Can you work these out from the drawing? Everything is in mm from the part's minimum corner. A direction names the side the tool comes from. Coordinates: 2 decimals unless noted, no trailing zeros. Order: outer loops, then holes, each group sorted by start corner. A loop starts at its lowest first (then second) coordinate and runs counter-clockwise, first axis right, second up. Notation, with made-up numbers: (76, -37) -> (134, -37) arc R9 cw to (134, -22) -> close; hole circle Ø4 at (89.5, -27). An arc over 180 degrees is marked (long way). Answer in a Markdown table with one row per item.
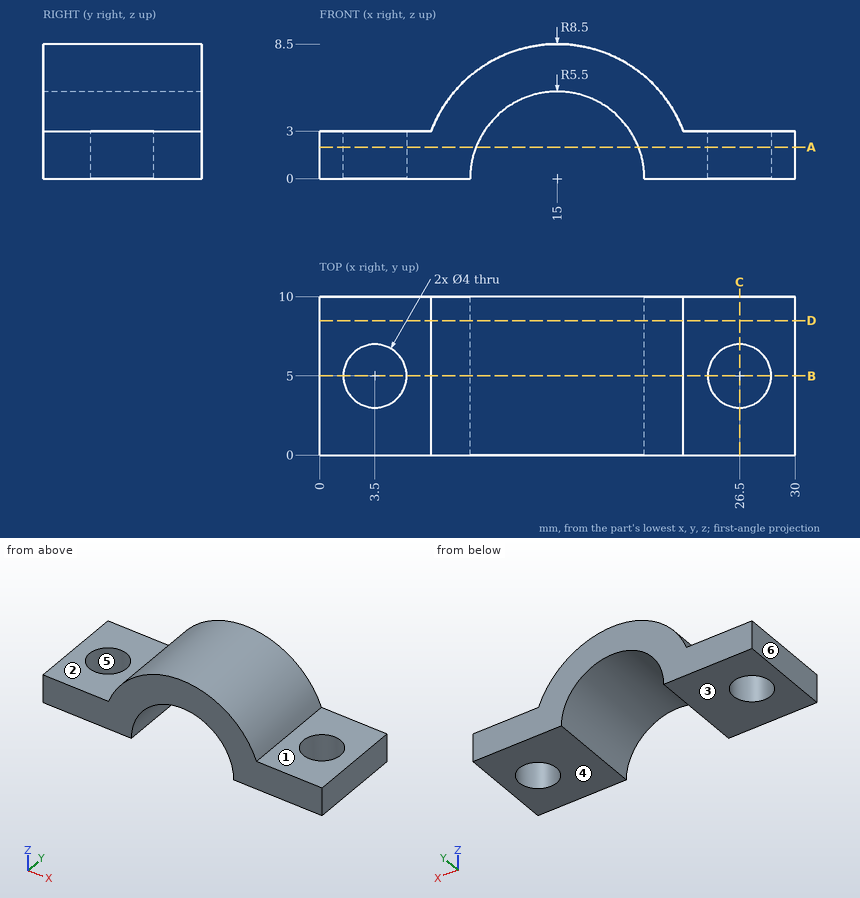
(1) Suppose I cut it at C-C (x = 26.5). Please give me the cut outline in (y, z), and give its area (3 significant figures).
Response values:
| item | result |
|---|---|
| outline | (0, 0) -> (3, 0) -> (3, 3) -> (0, 3) -> close; (7, 0) -> (10, 0) -> (10, 3) -> (7, 3) -> close |
| area | 18.0 mm2 |
(2) I need wall thicknesses on line 1 (Y direction, x = 26.5, z = 0.9); line 2 (X direction, y = 4.5, z = 1.75); line 3 (X direction, y = 6.25, z = 2.5). Which ranges of each line are inside material? Lowest first, please. Write a range as [from, to].
Response values:
| item | result |
|---|---|
| line 1 | [0, 3], [7, 10] |
| line 2 | [0, 1.56], [5.44, 9.79], [20.21, 24.56], [28.44, 30] |
| line 3 | [0, 1.94], [5.06, 10.1], [19.9, 24.94], [28.06, 30] |
(3) Suppose I cut it at A-A (z = 2). Please give me the cut outline in (x, y).
Response values:
| item | result |
|---|---|
| outline | (0, 0) -> (9.88, 0) -> (9.88, 10) -> (0, 10) -> close; (20.12, 0) -> (30, 0) -> (30, 10) -> (20.12, 10) -> close; hole circle Ø4 at (3.5, 5); hole circle Ø4 at (26.5, 5) |
(4) Suppose I cut it at D-D (y = 8.5). Please give me the cut outline in (x, z).
Response values:
| item | result |
|---|---|
| outline | (0, 0) -> (9.5, 0) arc R5.5 cw to (20.5, 0) -> (30, 0) -> (30, 3) -> (22.95, 3) arc R8.5 ccw to (7.05, 3) -> (0, 3) -> close |
(5) We'd pull the mould along X, two halves only. Please class the marked faces 4, 5 and 6: +X half, -X half, draft (parallel to the pull), parting line (faces both ways), or undercut.
Response values:
| item | result |
|---|---|
| face 4 | draft |
| face 5 | undercut |
| face 6 | -X half |
(6) Will these pins go through, and if not, where does the flat tip stop? pin 1 Ø6 at (x, y) = (6.5, 2) entering from +Z; pin 2 Ø3.5 at (x, y) = (27.5, 6) entering from +Z; pin 3 Ø3 at (x, y) = (6.5, 2) entering from +Z; pin 4 Ø3 at (x, y) = (3.5, 5) entering from +Z.
Response values:
| item | result |
|---|---|
| pin 1 | z = 6.48 |
| pin 2 | z = 3 |
| pin 3 | z = 4.82 |
| pin 4 | through |
(7) Suppose I cut it at B-B (y = 5). Please give me the cut outline in (x, z), and give its area (3 significant figures).
Response values:
| item | result |
|---|---|
| outline | (0, 0) -> (1.5, 0) -> (1.5, 3) -> (0, 3) -> close; (5.5, 0) -> (9.5, 0) arc R5.5 cw to (20.5, 0) -> (24.5, 0) -> (24.5, 3) -> (22.95, 3) arc R8.5 ccw to (7.05, 3) -> (5.5, 3) -> close; (28.5, 0) -> (30, 0) -> (30, 3) -> (28.5, 3) -> close |
| area | 82.1 mm2 |
(8) On a 3-axis mill with a long thin cutter (end or side, diameter ignored), from which of +Z, -Z, +X, -X, +Y, -Y can I reach the whole of each face in a straight line? I mean the marked faces 1, 2 and 3. Say none if no direction works.
Response values:
| item | result |
|---|---|
| face 1 | +Z, +X, +Y, -Y |
| face 2 | +Z, -X, +Y, -Y |
| face 3 | -Z, +X, -X, +Y, -Y |
